```python
from build123d import *

# Parameters (mm, degrees)
F1_DEPTH = 31.6
F2_START = 27.6
F2_DEPTH = 4
F0_R     = 3.05
F3_DEPTH = 2
F4_W     = 2.5
F4_H     = 29.6
F5_DEPTH = 2


with BuildPart() as f1:
    # F0 (on Top) → F1 (new body)
    with BuildSketch(Plane.XY):
        Polygon((31.25, -9), (31.25, 0), (29.25, 0), (29.25, -7), (-29.25, -7), (-29.25, 0), (-31.25, 0), (-31.25, -9), align=None)
        Polygon((31.25, 0), (31.25, 9), (-31.25, 9), (-31.25, 0), (-29.25, 0), (-29.25, 7), (29.25, 7), (29.25, 0), align=None)
    extrude(amount=F1_DEPTH)

    # F0 (on Top) → F2 (join)
    with BuildSketch(Plane.XY.offset(F2_START)):
        with BuildLine():
            Line((29, 0), (29.25, 0))
            Line((29.25, 0), (29.25, 7))
            Line((29.25, 7), (-29.25, 7))
            Line((-29.25, 7), (-29.25, 0))
            Line((-29.25, 0), (-29, 0))
            ThreePointArc((-29, 0), (-24.5, 4.5), (-20, 0))
            Line((-20, 0), (-16.1, 0))
            ThreePointArc((-16.1, 0), (-13.5, 2.6), (-10.9, 0))
            Line((-10.9, 0), (-7.1, 0))
            ThreePointArc((-7.1, 0), (-4.5, 2.6), (-1.9, 0))
            Line((-1.9, 0), (0, 0))
            Line((0, 0), (1.9, 0))
            ThreePointArc((1.9, 0), (4.5, 2.6), (7.1, 0))
            Line((7.1, 0), (10.9, 0))
            ThreePointArc((10.9, 0), (13.5, 2.6), (16.1, 0))
            Line((16.1, 0), (20, 0))
            ThreePointArc((20, 0), (24.5, 4.5), (29, 0))
        make_face()
        with BuildLine():
            Line((29.25, -7), (29.25, 0))
            Line((29.25, 0), (29, 0))
            ThreePointArc((29, 0), (24.5, -4.5), (20, 0))
            Line((20, 0), (16.1, 0))
            ThreePointArc((16.1, 0), (13.5, -2.6), (10.9, 0))
            Line((10.9, 0), (7.1, 0))
            ThreePointArc((7.1, 0), (4.5, -2.6), (1.9, 0))
            Line((1.9, 0), (0, 0))
            Line((0, 0), (-1.9, 0))
            ThreePointArc((-1.9, 0), (-4.5, -2.6), (-7.1, 0))
            Line((-7.1, 0), (-10.9, 0))
            ThreePointArc((-10.9, 0), (-13.5, -2.6), (-16.1, 0))
            Line((-16.1, 0), (-20, 0))
            ThreePointArc((-20, 0), (-24.5, -4.5), (-29, 0))
            Line((-29, 0), (-29.25, 0))
            Line((-29.25, 0), (-29.25, -7))
            Line((-29.25, -7), (29.25, -7))
        make_face()
    extrude(amount=F2_DEPTH)

    # F0 (on Top) → F3 (join)
    with BuildSketch(Plane.XY):
        Polygon((-41.25, 19), (-41.25, 14), (-41.25, -19), (41.25, -19), (41.25, 19), align=None)
        with Locations((-27.5, 14)):
            Circle(F0_R, mode=Mode.SUBTRACT)
        Polygon((-31.25, 9), (31.25, 9), (31.25, 0), (31.25, -9), (-31.25, -9), (-31.25, 0), align=None, mode=Mode.SUBTRACT)
        with Locations((27.5, 14)):
            Circle(F0_R, mode=Mode.SUBTRACT)
    extrude(amount=F3_DEPTH)

    # F4 (on face) → F5 (cut)
    with BuildSketch(Plane.XZ.offset(9)):
        with Locations((-1.25, 16.8)):
            Rectangle(F4_W, F4_H)
        with Locations((1.25, 16.8)):
            Rectangle(F4_W, F4_H)
        with Locations((-19.25, 16.8)):
            Rectangle(F4_W, F4_H)
        with Locations((-16.75, 16.8)):
            Rectangle(F4_W, F4_H)
        with Locations((-10.25, 16.8)):
            Rectangle(F4_W, F4_H)
        with Locations((-7.75, 16.8)):
            Rectangle(F4_W, F4_H)
        with Locations((10.25, 16.8)):
            Rectangle(F4_W, F4_H)
        with Locations((7.75, 16.8)):
            Rectangle(F4_W, F4_H)
        with Locations((16.75, 16.8)):
            Rectangle(F4_W, F4_H)
        with Locations((19.25, 16.8)):
            Rectangle(F4_W, F4_H)
    extrude(amount=-F5_DEPTH, mode=Mode.SUBTRACT)


solid = f1.part
```
Source: CAD feature listing. Evaluate the final solid. Frame: model axes, mm. A direction names the side the tool comes from. Give positions to 0.01 mm unless a question says otherwise; leave off trailing zeros. Loops run counter-clockwise (first coordinate to the right, second up) from the corner with the lowest first, then second, coordinate; pieces in that order, holes last. Notation, with made-up numbers: (-29, 84) -> (-21, 84) arc R19 ccw to (-21, 94) -> close; hole circle Ø5 at (54, 11.5). An arc over 180 degrees is marked (long way). Use a Markdown table: item, result. Add a question column.
(1) Pull-direction query (X, two-part tool) for faces 1 (the face through (31.25, 0, 17)), 2 (the face through (20.5, -8, 17)), 3 (the face through (0, 9, 17)), 4 (the face through (15.98, -0.78, 29.57)); classes: +X half, -X half, draft (parallel to the pull), parting line (faces both ways), or undercut.
(2) Section query A-A (z = 13.5). Output: boundary loops of the cut face in (x, y).
(3) Access query for faces 5 (the face through (18, -7, 30)), 6 (the face through (-31.25, 0, 17)), 7 (the face through (-41.25, 0, 1)). Directions: +Z, -Z, +X, -X, +Y, -Y. A direction counts if a zero-diameter tool reaches every point of the face in a straight line with its end or side. Return the directions, or none.
(4) First-contact query: pin 1 Ø2 at (x, y) = (-2.5, 14) entering from +Z; pin 2 Ø1 at (y, z) = (3, 25.5) entering from -X; pin 3 Ø6 at (x, z) = (-2, 22.5) entering from -Y; pin 4 Ø6 at (x, y) = (4.5, 0) entering from +Z. Flat tips, straight axial feed; report the tip coordinate or a pass-through.
(5) Section query D-D (x = 27.5). Output: boundary loops of the cut face in (y, z).
(6) Ray query, line 1 (Y direction, x = -15, z = 8); line 2 (X direction, y = 4, z = 13); line 3 (Z direction, x = -15, y = 14). Return the intervals inside material, ascending.
(7) Section query B-B (y = 14). Output: boundary loops of the cut face in (x, z).
(8) Section query C-C (x = -5.5). Output: boundary loops of the cut face in (y, z).
Checked values:
| question | item | result |
|---|---|---|
| 1 | face 1 | +X half |
| 1 | face 2 | undercut |
| 1 | face 3 | draft |
| 1 | face 4 | undercut |
| 2 | outline | (-31.25, -9) -> (-20.5, -9) -> (-20.5, -7) -> (-29.25, -7) -> (-29.25, 7) -> (29.25, 7) -> (29.25, -7) -> (20.5, -7) -> (20.5, -9) -> (31.25, -9) -> (31.25, 9) -> (-31.25, 9) -> close; (-15.5, -9) -> (-11.5, -9) -> (-11.5, -7) -> (-15.5, -7) -> close; (-6.5, -9) -> (-2.5, -9) -> (-2.5, -7) -> (-6.5, -7) -> close; (2.5, -9) -> (6.5, -9) -> (6.5, -7) -> (2.5, -7) -> close; (11.5, -9) -> (15.5, -9) -> (15.5, -7) -> (11.5, -7) -> close |
| 3 | face 5 | +Z, -Y |
| 3 | face 6 | +Z, -X, +Y, -Y |
| 3 | face 7 | +Z, -Z, -X, +Y, -Y |
| 4 | pin 1 | z = 2 |
| 4 | pin 2 | x = -31.25 |
| 4 | pin 3 | y = -9 |
| 4 | pin 4 | z = 31.6 |
| 5 | outline | (-19, 0) -> (-7, 0) -> (-7, 27.6) -> (-3.35, 27.6) -> (-3.35, 31.6) -> (-9, 31.6) -> (-9, 2) -> (-19, 2) -> close; (3.35, 27.6) -> (7, 27.6) -> (7, 0) -> (10.95, 0) -> (10.95, 2) -> (9, 2) -> (9, 31.6) -> (3.35, 31.6) -> close; (17.05, 0) -> (19, 0) -> (19, 2) -> (17.05, 2) -> close |
| 6 | line 1 | -9 to -7, 7 to 9 |
| 6 | line 2 | -31.25 to -29.25, 29.25 to 31.25 |
| 6 | line 3 | 0 to 2 |
| 7 | outline | (-41.25, 0) -> (-30.55, 0) -> (-30.55, 2) -> (-41.25, 2) -> close; (-24.45, 0) -> (24.45, 0) -> (24.45, 2) -> (-24.45, 2) -> close; (30.55, 0) -> (41.25, 0) -> (41.25, 2) -> (30.55, 2) -> close |
| 8 | outline | (-19, 0) -> (-7, 0) -> (-7, 27.6) -> (-2.4, 27.6) -> (-2.4, 31.6) -> (-9, 31.6) -> (-9, 2) -> (-19, 2) -> close; (2.4, 27.6) -> (7, 27.6) -> (7, 0) -> (19, 0) -> (19, 2) -> (9, 2) -> (9, 31.6) -> (2.4, 31.6) -> close |
